Work out the finished part from the listing and answer in its coordinate system (mm). A direction names the side the tool comes from. Round coordinates to 2 decimals unless told otherwise and drop trailing zeros. Order: outer loops, then holes, each group sorted by start corner. A loop starts at its lowest first (then second) coordinate and runs counter-clockwise, first axis right, second up. Notation, with made-up numbers: (-25, -25) - (-15, -25) arc R9 cw to (-15, -19) - close; hole circle Ø3 at (28.5, 71.25). An arc over 180 degrees is marked (long way). Use CSV: the item, a comma, the result in double quotes.
Autodesk Inventor part; units mm, degrees
ref_plane "YZ Plane" through (0, 0, 0) normal (1, 0, 0) x (0, 1, 0)
ref_plane "XZ Plane" through (0, 0, 0) normal (0, 1, 0) x (-1, 0, 0)
ref_plane "XY Plane" through (0, 0, 0) normal (0, 0, 1) x (1, 0, 0)
sketch "Szkic1" plane through (0, 0, 0) normal (1, 0, 0) x (0, 1, 0)
  line L0 (13.7, -0.2) -> (25.3, -0.2)
  line L1 (13.5, 0) -> (13.7, -0.2)
  line L2 (0, 0) -> (13.5, 0)
  line L3 (-0.5, -0.5) -> (0, 0)
  line L4 (-0.5, -3.7085) -> (-0.5, -0.5)
  arc A0 (-0.783, -4.008) -> (-0.5, -3.7085) centre (-0.8, -3.7085) ccw
  arc A1 (-0.783, -4.008) -> (3.9514, -6.7229) centre (-0.5, -9) ccw
  arc A2 (4.0685, -6.3265) -> (3.9514, -6.7229) centre (4.2185, -6.5863) ccw
  line L5 (5.5, -5.5) -> (4.0685, -6.3265)
  line L6 (19, -5.5) -> (5.5, -5.5)
  line L7 (19.5, -5.2113) -> (19, -5.5)
  line L8 (20, -5.5) -> (19.5, -5.2113)
  line L9 (33.5, -5.5) -> (20, -5.5)
  line L10 (34.9315, -6.3265) -> (33.5, -5.5)
  arc A3 (35.0486, -6.7229) -> (34.9315, -6.3265) centre (34.7815, -6.5863) ccw
  arc A4 (35.0486, -6.7229) -> (39.783, -4.008) centre (39.5, -9) ccw
  arc A5 (39.5, -3.7085) -> (39.783, -4.008) centre (39.8, -3.7085) ccw
  line L11 (39.5, -0.5) -> (39.5, -3.7085)
  line L12 (39, 0) -> (39.5, -0.5)
  line L13 (25.5, 0) -> (39, 0)
  line L14 (25.3, -0.2) -> (25.5, 0)
  point P0 (19.5, 0)
extrude "Wyciągnięcie proste1" add sketch "Szkic1" along normal blind 50
properties part number "WS_10_40_custom_length"
(1) Find section C-C (y = 9). Determine the outline of the cut face in (x, z).
Findings below:
outline,"(0, -5.5) - (50, -5.5) - (50, 0) - (0, 0) - close"
(2) Find the intervals of material crossed by L1, parallel to Y at x = 23, z = -1.5; L2, parallel to Z at x = 9.5, y = 9; L3, parallel to Y at x = 47, z = -10.75, in increasing order. Write a range as from..to.
Findings below:
L1,"y = -0.5..39.5"
L2,"z = -5.5..0"
L3,"y = -5.18..4.18, 34.82..44.18"
(3) Find section D-D (y = 16). Determine the outline of the cut face in (x, z).
Findings below:
outline,"(0, -5.5) - (50, -5.5) - (50, -0.2) - (0, -0.2) - close"
(4) Find section B-B (x = 6). Determine the outline of the cut face in (y, z), and give its area (3 significant figures).
Findings below:
outline,"(-0.78, -4.01) arc R5 ccw (long way) to (3.95, -6.72) arc R0.3 cw to (4.07, -6.33) - (5.5, -5.5) - (19, -5.5) - (19.5, -5.21) - (20, -5.5) - (33.5, -5.5) - (34.93, -6.33) arc R0.3 cw to (35.05, -6.72) arc R5 ccw (long way) to (39.78, -4.01) arc R0.3 cw to (39.5, -3.71) - (39.5, -0.5) - (39, 0) - (25.5, 0) - (25.3, -0.2) - (13.7, -0.2) - (13.5, 0) - (0, 0) - (-0.5, -0.5) - (-0.5, -3.71) arc R0.3 cw to start"
area,"369 mm²"
(5) For faces 1 (the flat face through (25, 12, -5.5)), 2 (the flat face through (24.65, 34.23, -5.92)), 3 (the flat face through (25, 39.5, -2)), determine the directions among +Z, -Z, +X, -X, +Y, -Y from which every point of the face is accessible in a straight line to the end or side of a thin tool.
Findings below:
face 1,"-Z, +X, -X"
face 2,"+X, -X"
face 3,"+Z, +X, -X, +Y"
(6) Each of these flat-tipped pins is pushed along its axis until it touches: pin 1 (1 mm diameter, centred on x = 16, z = -2.5, fed in from +Y); pin 2 (6 mm diameter, centred on x = 14, y = 18.5, fed in from +Z); pin 3 (7 mm diameter, centred on x = 32.5, y = 11.5, fed in from -Z); pin 4 (6 mm diameter, centred on y = 39, z = -11.5, fed in from -X). Where does it stop, or does it pass through?
Findings below:
pin 1,"stops at y = 39.5"
pin 2,"stops at z = -0.2"
pin 3,"stops at z = -5.5"
pin 4,"stops at x = 0"
(7) Find section A-A (z = -9). Determine the outline of the cut face in (x, y), and give its area (3 significant figures).
Findings below:
outline,"(0, -5.5) - (50, -5.5) - (50, 4.5) - (0, 4.5) - close; (0, 34.5) - (50, 34.5) - (50, 44.5) - (0, 44.5) - close"
area,"1,000 mm²"
